Build history of the part. All positions in model axes, mm. Face numbers are marked on the shaded views. Round coordinates to 2 decimals unless told otherwise and drop trailing zeros. Order: outer loops, then holes, each group sorted by start corner. A loop starts at its lowest first (then second) coordinate and runs counter-clockwise, first axis right, second up. Notation, with made-up numbers: (37.25, 17.5) -> (41.25, 17.5) arc R9 cw to (41.25, 33.5) -> close; hole circle Ø8 at (36, -11.5). An arc over 180 degrees is marked (long way). Use a Markdown table: item, result. Add a question column.
Item 1: Slice it at D-D, the plane x = 29.5. Give the cut face in (y, z).
Item 2: Slice it at B-B, the plane x = -39. Give the cut face in (y, z), plus the area to 3 significant figures.
Item 3: Two-plate mould, pull along Y, no slides. Class the marked faces 1, 2, 3 and 4: released by +Y, released by -Y, zero draft, split by the parting line, or undercut.
Item 4: Slice it at A-A, the plane z = 177.5. Give the cut face in (x, y), plus the area to 3 significant figures.
Item 5: Probe L1, parallel to Z at x = -90.5, y = -61; L2, parallel to Z at x = 32, y = -30; L3, parallel to X at y = -55.5, z = 30.5. List the from-to ranges inside material, lowest first.
Item 6: Pin check, flat tips, straight feed: pin 1 (5.5 mm diameter, centred on x = 44.5, z = 223.5, fed in from +Y); pin 2 (6 mm diameter, centred on x = 7, y = -52.5, fed in from +Z); pin 3 (10.5 mm diameter, centred on y = -23.5, z = 196, fed in from -X); pin 4 (8 mm diameter, centred on x = -41, y = -67, fed in from +Z). Stop position of each tip, or through.
Item 7: Slice it at C-C, the plane y = -59. Give the cut face in (x, z), plus the area to 3 significant figures.
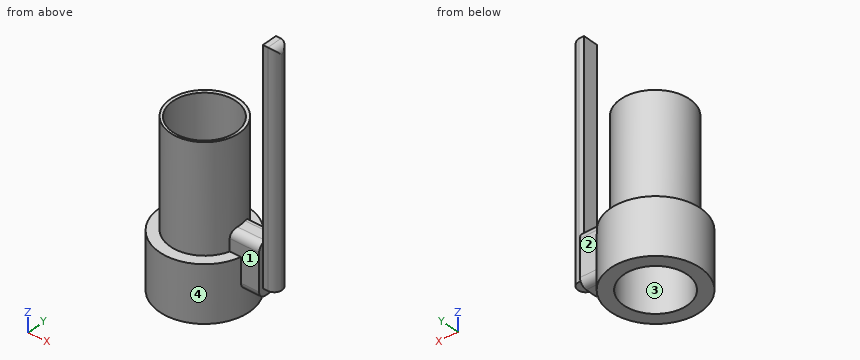
from build123d import *

# Parameters (mm, degrees)
F0_R      = 47.117
F1_DEPTH  = 220.98
F3_D      = 78.74
F4_R      = 61.2968374211
F5_DEPTH  = 76.2
F7_D      = 86.36
F8_W      = 33.8315991685
F8_H      = 70.290889591
F9_DEPTH  = 40.894
F10_R     = 10.16
F11_W     = 21.0215765983
F11_H     = 1.9707717001
F12_DEPTH = 17.018
F13_W     = 17.018
F13_H     = 21.0215765983
F14_DEPTH = 308.61
F15_R     = 10.16


with BuildPart() as f1:
    # F0 (on Top) → F1 (new body)
    with BuildSketch(Plane.XY):
        with Locations((-44.1687442362, -30.721032992)):
            Circle(F0_R)
    extrude(amount=F1_DEPTH)

    # F3 (through all)
    with Locations(Plane(origin=(0, 0, 0), x_dir=(1, 0, 0), z_dir=(0, 0, -1))):
        with Locations((-44.1687442362, 30.721032992)):
            Hole(F3_D / 2)

    # F4 (on Top) → F5 (join)
    with BuildSketch(Plane.XY):
        with Locations((-43.806668371, -31.8049825728)):
            Circle(F4_R)
    extrude(amount=F5_DEPTH)

    # F7 (through all)
    with Locations(Plane(origin=(0, 0, 0), x_dir=(1, 0, 0), z_dir=(0, 0, -1))):
        with Locations((-43.806668371, 31.8049825728)):
            Hole(F7_D / 2)

    # F8 (on Right) → F9 (join)
    with BuildSketch(Plane.YZ):
        with Locations((-27.3374826647, 67.7915308625)):
            Rectangle(F8_W, F8_H)
    extrude(amount=F9_DEPTH)

    # F10
    f10_edges = [f1.edges().sort_by_distance(p)[0] for p in [
        (20.447, -10.421683, 102.936976),
        (20.928586, -44.253282, 102.936976),
        (27.266726, -10.421683, 32.646086),
        (28.553423, -44.253282, 32.646086),
    ]]
    fillet(f10_edges, radius=F10_R)

    # F11 (on face) → F12 (join)
    with BuildSketch(Plane.YZ.offset(40.894)):
        with Locations((-27.5017125532, 44.7991844267)):
            Rectangle(F11_W, F11_H)
    extrude(amount=F12_DEPTH)

    # F13 (on face) → F14 (join)
    with BuildSketch(Plane.XY.offset(45.7845702767)):
        with Locations((49.403, -27.5017125532)):
            Rectangle(F13_W, F13_H)
    extrude(amount=F14_DEPTH)

    # F15
    f15_edges = [f1.edges().sort_by_distance(p)[0] for p in [
        (57.912, -38.012501, 199.104184),
        (57.912, -16.990924, 199.104184),
        (57.912, -27.501713, 354.39457),
    ]]
    fillet(f15_edges, radius=F15_R)


solid = f1.part
Check sheet entries:
| question | item | result |
|---|---|---|
| 1 | outline | (-44.25, 42.81) arc R10.16 ccw to (-34.09, 32.65) -> (-20.58, 32.65) arc R10.16 ccw to (-10.42, 42.81) -> (-10.42, 92.78) arc R10.16 ccw to (-20.58, 102.94) -> (-34.09, 102.94) arc R10.16 ccw to (-44.25, 92.78) -> close |
| 2 | outline | (-92.91, 0) -> (-74.72, 0) -> (-74.72, 220.98) -> (-77.55, 220.98) -> (-77.55, 76.2) -> (-92.91, 76.2) -> close; (11.11, 0) -> (29.3, 0) -> (29.3, 76.2) -> (16.11, 76.2) -> (16.11, 220.98) -> (11.11, 220.98) -> close |
| 2 | area | 3,910 mm2 |
| 3 | face 1 | released by -Y |
| 3 | face 2 | released by +Y |
| 3 | face 3 | undercut |
| 3 | face 4 | split by the parting line |
| 4 | outline | circle Ø94.23 at (-44.17, -30.72); (40.89, -38.01) -> (47.75, -38.01) arc R10.16 ccw to (57.91, -27.85) -> (57.91, -27.15) arc R10.16 ccw to (47.75, -16.99) -> (40.89, -16.99) -> close; hole circle Ø86.36 at (-43.81, -31.8) |
| 4 | area | 1,430 mm2 |
| 5 | L1 | 0 to 76.2 |
| 5 | L2 | 32.65 to 102.94 |
| 5 | L3 | -100.34 to -79.9, -7.71 to 12.73 |
| 6 | pin 1 | y = -16.99 |
| 6 | pin 2 | z = 76.2 |
| 6 | pin 3 | x = -91.24 |
| 6 | pin 4 | through |
| 7 | outline | (-98.74, 0) -> (-77.35, 0) -> (-77.35, 220.98) -> (-81.86, 220.98) -> (-81.86, 76.2) -> (-98.74, 76.2) -> close; (-10.27, 0) -> (11.13, 0) -> (11.13, 76.2) -> (-6.48, 76.2) -> (-6.48, 220.98) -> (-10.27, 220.98) -> close |
| 7 | area | 4,460 mm2 |
